Model file for the job. Use its own axes, mm. A direction names the side the tool comes from. Give positions to 0.01 mm unless a question says otherwise; leave off trailing zeros. Write each loop counter-clockwise with the first axis right and the second up, starting at its lowest first coordinate (ties: lowest second). Pieces come first, ordered by that corner, then holes. Notation, with made-up numbers: (64.5, 33) - (109.5, 33) arc R9 cw to (109.5, 39) - close; hole circle Ø10 at (-30, 16). An arc over 180 degrees is marked (long way). Use a Markdown table: item, result. Add a question column.
```python
from build123d import *

# Parameters (mm, degrees)
ESQUISSE2_W            = 33.813849949
ESQUISSE2_H            = 50.207047895
BOSS_EXTRU_1_DEPTH     = 4.5
ESQUISSE6_W            = 26.70455913
ESQUISSE6_H            = 28.958
BOSS_EXTRU_ASICS_DEPTH = 1.5
ESQUISSE7_R            = 3
BOSS_EXTRU_FIXS_DEPTH  = 3.5
TROU_TARAUD_M31_D      = 2.5
TROU_TARAUD_M31_DEPTH  = 8


with BuildPart() as part:
    # Esquisse2 → Boss.-Extru.1 (new body)
    with BuildSketch(Plane.XY):
        with Locations((97.906924975, -94.896476053)):
            Rectangle(ESQUISSE2_W, ESQUISSE2_H)
    extrude(amount=BOSS_EXTRU_1_DEPTH)

    # Esquisse6 → Boss.-Extru. ASICs (add)
    with BuildSketch(Plane(origin=(0, 0, 0), x_dir=(-1, 0, 0), z_dir=(0, 0, -1))):
        with Locations((-98.850279565, -94.521)):
            Rectangle(ESQUISSE6_W, ESQUISSE6_H)
    extrude(amount=BOSS_EXTRU_ASICS_DEPTH)

    # Esquisse7 → Boss.-Extru. FIXs (add)
    with BuildSketch(Plane(origin=(0, 0, 0), x_dir=(-1, 0, 0), z_dir=(0, 0, -1))):
        with Locations((-86, -74)):
            Circle(ESQUISSE7_R)
        with Locations((-86, -115)):
            Circle(ESQUISSE7_R)
    extrude(amount=BOSS_EXTRU_FIXS_DEPTH)

    # Trou taraudé M31
    with Locations(Plane(origin=(0, 0, -3.5), x_dir=(-1, 0, 0), z_dir=(0, 0, -1))):
        with Locations((-86, -74), (-86, -115)):
            Hole(TROU_TARAUD_M31_D / 2, depth=TROU_TARAUD_M31_DEPTH)


solid = part.part
```
(1) Band-saw the part on B-B (y = -115). Write the cut outline in (x, z).
(2) Band-saw the part on D-D (x = 96.5). Write the cut outline in (y, z), then the cut area to 3 significant figures.
(3) Band-saw the part on A-A (z = -0.5). Write the cut outline in (x, y).
(4) Which spindle directions (+Z, -Z, +X, -X, +Y, -Y) get a long thin tool onto all of the face, cutting with end or side? Do faces 5 (the flat face through (112.203, -95, -1)), 6 (the cylindrical face through (88.4, -75.8, -1.7)), 7 (the flat face through (114.814, -95, 2)). Say none if no direction does.
(5) Probe probe 1 along Y at (x, z) = (86, 0.75); probe 2 along Y at (x, z) = (86, -0.25); probe 3 along X at (y, z) = (-115, 0.25). List the from-to ranges inside material, lowest first. Write a range as [from, to].
(6) Two-plate mould, pull along Y, no slides. Class faces 1 (the flat face through (98, -120, 2)), 2 (the cylindrical face through (88.21, -112.97, -1.73)), 3 (the flat face through (85, -75, -3.5)), 4 (the flat face through (85.498, -95, -1)): +Y half, -Y half, draft (parallel to the pull), parting line (faces both ways), or undercut.
(7) Band-saw the part on C-C (x = 86). Write the cut outline in (y, z).
(8) Flat gauge pins, fed straight in: pin 1 (8 mm diameter, centred on x = 103, y = -88, fed in from -Z); pin 2 (1.6 mm diameter, centred on x = 102, z = -0.5, fed in from -Y); pin 3 (3 mm diameter, centred on y = -99.5, z = -2, fed in from -X); pin 4 (2 mm diameter, centred on x = 86, y = -74, fed in from -Z). Where does each tip first touch, or does it go through?
Model answer:
| question | item | result |
|---|---|---|
| 1 | outline | (81, 0) - (83, 0) - (83, -3.5) - (84.75, -3.5) - (84.75, 4.5) - (81, 4.5) - close; (87.25, -3.5) - (89, -3.5) - (89, 0) - (114.81, 0) - (114.81, 4.5) - (87.25, 4.5) - close |
| 2 | outline | (-120, 0) - (-109, 0) - (-109, -1.5) - (-80.04, -1.5) - (-80.04, 0) - (-69.79, 0) - (-69.79, 4.5) - (-120, 4.5) - close |
| 2 | area | 269 mm^2 |
| 3 | outline | circle Ø6 at (86, -115); circle Ø6 at (86, -74); (85.5, -109) - (112.2, -109) - (112.2, -80.04) - (85.5, -80.04) - close; hole circle Ø2.5 at (86, -115); hole circle Ø2.5 at (86, -74) |
| 4 | face 5 | -Z, +X, +Y, -Y |
| 4 | face 6 | -Z |
| 4 | face 7 | +Z, -Z, +X, +Y, -Y |
| 5 | probe 1 | y = [-120, -116.25], [-113.75, -75.25], [-72.75, -69.79] |
| 5 | probe 2 | y = [-118, -116.25], [-113.75, -112], [-109, -80.04], [-77, -75.25], [-72.75, -71] |
| 5 | probe 3 | x = [81, 84.75], [87.25, 114.81] |
| 6 | face 1 | -Y half |
| 6 | face 2 | undercut |
| 6 | face 3 | draft |
| 6 | face 4 | undercut |
| 7 | outline | (-120, 0) - (-118, 0) - (-118, -3.5) - (-116.25, -3.5) - (-116.25, 4.5) - (-120, 4.5) - close; (-113.75, -3.5) - (-112, -3.5) - (-112, 0) - (-109, 0) - (-109, -1.5) - (-80.04, -1.5) - (-80.04, 0) - (-77, 0) - (-77, -3.5) - (-75.25, -3.5) - (-75.25, 4.5) - (-113.75, 4.5) - close; (-72.75, -3.5) - (-71, -3.5) - (-71, 0) - (-69.79, 0) - (-69.79, 4.5) - (-72.75, 4.5) - close |
| 8 | pin 1 | stops at z = -1.5 |
| 8 | pin 2 | stops at y = -120 |
| 8 | pin 3 | stops at x = 85.5 |
| 8 | pin 4 | passes through |
